```python
from build123d import *

# Parameters (mm, degrees)
F0_R     = 8.75
F0_R_2   = 6.05
F0_R_3   = 5
F1_DEPTH = 20
F0_R_4   = 3.75
F2_DEPTH = 10
F0_R_5   = 2.65
F3_DEPTH = 6.2
F5_DEPTH = 10
F6_DEPTH = 6.5


with BuildPart() as f1:
    # F0 (on Top) → F1 (new body)
    with BuildSketch(Plane.XY):
        Circle(F0_R)
        Circle(F0_R_2, mode=Mode.SUBTRACT)
        Circle(F0_R_2)
        Circle(F0_R_3, mode=Mode.SUBTRACT)
    extrude(amount=F1_DEPTH)

    # F4 (on face) → F5 (cut)
    with BuildSketch(Plane.XY.offset(20)):
        with BuildLine():
            ThreePointArc((-5.8576872569, -6.5), (0, -8.75), (5.8576872569, -6.5))
            Line((5.8576872569, -6.5), (-5.8576872569, -6.5))
        make_face()
        with BuildLine():
            Line((-5.8576872569, 6.5), (5.8576872569, 6.5))
            ThreePointArc((5.8576872569, 6.5), (0, 8.75), (-5.8576872569, 6.5))
        make_face()
    extrude(amount=-F5_DEPTH, mode=Mode.SUBTRACT)



with BuildPart() as f2:
    # F0 (on Top) → F2 (new body)
    with BuildSketch(Plane.XY):
        Circle(F0_R_3)
        Circle(F0_R_4, mode=Mode.SUBTRACT)
    extrude(amount=F2_DEPTH)

    # F0 (on Top) → F3 (join)
    with BuildSketch(Plane.XY):
        Circle(F0_R_4)
        Circle(F0_R_5, mode=Mode.SUBTRACT)
    extrude(amount=F3_DEPTH)


with BuildPart() as f1_1:
    add(f1.part)

    add(f2.part)  # F6 merges F2
    # F0 (on Top) → F6 (join)
    with BuildSketch(Plane.XY):
        Circle(F0_R_2)
        Circle(F0_R_3, mode=Mode.SUBTRACT)
        Circle(F0_R_3)
        Circle(F0_R_4, mode=Mode.SUBTRACT)
        Circle(F0_R_4)
        Circle(F0_R_5, mode=Mode.SUBTRACT)
    extrude(amount=-F6_DEPTH)


solid = f1_1.part
```
The model under review builds one solid part; all positions refer to its coordinate system, in mm. A direction names the side the tool comes from. Round coordinates to 2 decimals unless told otherwise and drop trailing zeros. Write each loop counter-clockwise with the first axis right and the second up, starting at its lowest first coordinate (ties: lowest second). Pieces come first, ordered by that corner, then holes.
(1) Mouldability with a two-part tool opening along X and no side actions: class faces 5 (the cylindrical face through (5.589, -2.317, -3.204)), 6 (the flat face through (3, -1, -6.5)), 7 (the flat face through (1, 3, 6.2)) as +X half, -X half, draft (parallel to the pull), parting line (faces both ways), or undercut.
(2) We need section C-C on x = 1.75. Give the boundary of the cut face in (y, z), and give its area (3 significant figures).
(3) We need section B-B on z = 14.25. Give the boundary of the cut face in (x, y).
(4) Machinability: for faces 1 (the flat face through (0, 7, 10)), 2 (the cylindrical face through (-3.746, 0.165, 8.073)), 3 (the flat face through (0, -6.5, 15)), 4 (the flat face through (-2, -6, 0)), which of the approach directions +Z, -Z, +X, -X, +Y, -Y give a long, thin tool a straight path to every point of the face, cutting with its end or side? Answer none if there is none.
(5) Insertion check: pin 1 (8.5 mm diameter, centred on x = 0, y = 0, fed in from +Z); pin 2 (4 mm diameter, centred on x = 0, y = 0, fed in from -Z) (3 decimals); pin 3 (6 mm diameter, centred on x = 0, y = 0, fed in from +Z); pin 4 (2 mm diameter, centred on x = -4.5, z = 6, fed in from -Y). Each pin has a flat end and moves straight along its axis. Give the tip position at first contact, or say it passes through.
(6) We need section D-D on x = -4.25. Give the boundary of the cut face in (y, z), and give its area (3 significant figures).
(7) We need section A-A on x = 0. Give the boundary of the cut face in (y, z), and give its area (3 significant figures).
(8) Wall thickness on L1, parallel to Y at x = 0, z = 9.25; L2, parallel to Y at x = 0, z = 17; L3, parallel to X at y = 0.25, z = 14.5: over which ranges is each line inside the solid? List them lowest first.
Findings below:
1. face 5: parting line
1. face 6: draft
1. face 7: undercut
2. outline: (-8.57, 0) - (-5.79, 0) - (-5.79, -6.5) - (-1.99, -6.5) - (-1.99, 6.2) - (-3.32, 6.2) - (-3.32, 10) - (-4.68, 10) - (-4.68, 20) - (-6.5, 20) - (-6.5, 10) - (-8.57, 10) - close; (1.99, -6.5) - (5.79, -6.5) - (5.79, 0) - (8.57, 0) - (8.57, 10) - (6.5, 10) - (6.5, 20) - (4.68, 20) - (4.68, 10) - (3.32, 10) - (3.32, 6.2) - (1.99, 6.2) - close
2. area: 207 mm2
3. outline: (-5.86, -6.5) - (5.86, -6.5) arc R8.75 ccw to (5.86, 6.5) - (-5.86, 6.5) arc R8.75 ccw to start; hole circle Ø10 at (0, 0)
4. face 1: +Z, +X, -X, +Y
4. face 2: +Z
4. face 3: +Z, +X, -X, -Y
4. face 4: -Z
5. pin 1: stops at z = 10
5. pin 2: passes through
5. pin 3: stops at z = 6.2
5. pin 4: stops at y = -8.02
6. outline: (-7.65, 0) - (-4.31, 0) - (-4.31, -6.5) - (4.31, -6.5) - (4.31, 0) - (7.65, 0) - (7.65, 10) - (6.5, 10) - (6.5, 20) - (2.63, 20) - (2.63, 10) - (-2.63, 10) - (-2.63, 20) - (-6.5, 20) - (-6.5, 10) - (-7.65, 10) - close
6. area: 286 mm2
7. outline: (-8.75, 0) - (-6.05, 0) - (-6.05, -6.5) - (-2.65, -6.5) - (-2.65, 6.2) - (-3.75, 6.2) - (-3.75, 10) - (-5, 10) - (-5, 20) - (-6.5, 20) - (-6.5, 10) - (-8.75, 10) - close; (2.65, -6.5) - (6.05, -6.5) - (6.05, 0) - (8.75, 0) - (8.75, 10) - (6.5, 10) - (6.5, 20) - (5, 20) - (5, 10) - (3.75, 10) - (3.75, 6.2) - (2.65, 6.2) - close
7. area: 188 mm2
8. L1: y = -8.75 to -3.75, 3.75 to 8.75
8. L2: y = -6.5 to -5, 5 to 6.5
8. L3: x = -8.75 to -4.99, 4.99 to 8.75
